Study the drawing (mm; zero at the part's minimum x, y, z) and answer. Give positions to 0.01 mm unless a question says otherwise; leave off trailing zeros. Write each loop counter-clockwise with the first axis right and the second up, starting at its lowest first coordinate (ties: lowest second). Pieces come first, ordered by that corner, then holes. Notation, with made-up numbers: (-19.75, 72) -> (-10.75, 72) arc R18 ccw to (-10.75, 104) -> close; hole circle Ø6 at (-35, -25.75). An arc over 180 degrees is marked (long way). Use CSV: the item, a comma, the result in double quotes. Start each with the question number.
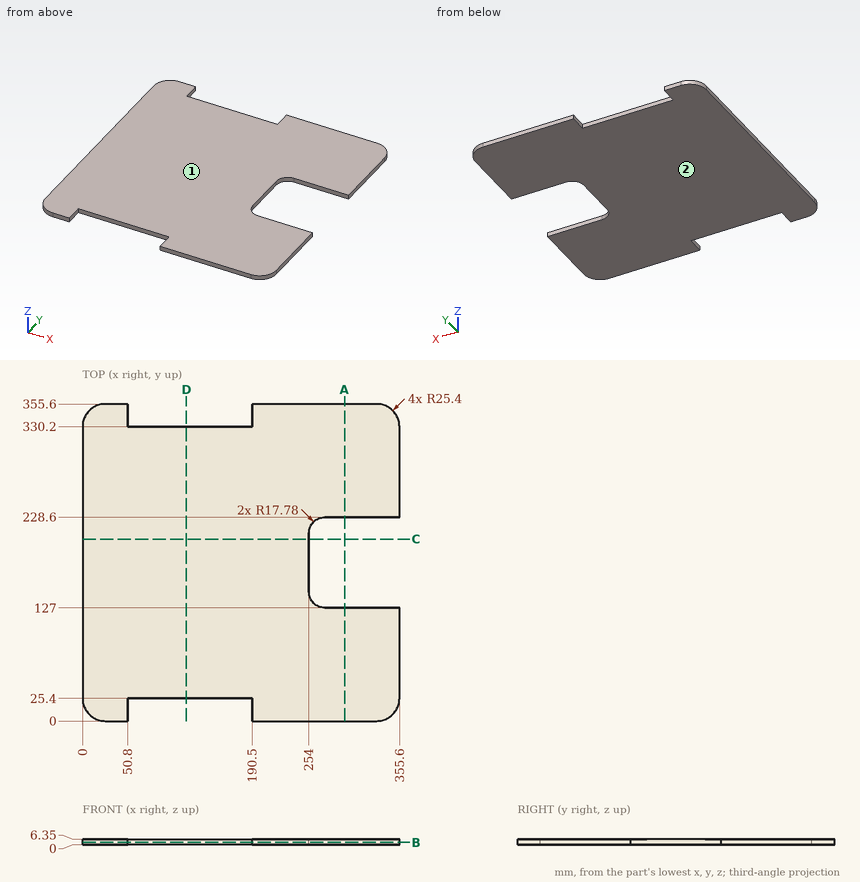
Q1. Section B-B on z = 2.5 is taken. Give the vertices of the cut face in (x, y).
Q2. Straight lines are drawn through the part: L1, parallel to Y at x = 284, z = 5.25; L2, parallel to Y at x = 88, z = 0.5; L3, parallel to X at y = 182.5, z = 4. For each, find the intervals that lie inside material, in ascending order.
Q3. Section D-D on x = 116.5 is taken. Give the vertices of the cut face in (y, z).
Q4. Flat-ended cylindrical pins translate along their axes: pin 1 Ø3 at (y, z) = (13, 3) entering from +X; pin 2 Ø1.9 at (y, z) = (342, 2.5) entering from +X; pin 3 Ø1 at (x, z) = (84, 3.5) entering from +Y. Find the tip coordinate at first contact, or state that the pin passes through.
Q5. Section A-A on x = 294 is taken. Give the vertices of the cut face in (y, z).
Q6. The mould has two halves that part along Z. Classify the marked faces 1 and 2: +Z half, -Z half, draft (parallel to the pull), parting line (faces both ways), or undercut.
Q7. Section C-C on y = 204 is taken. Give the vertices of the cut face in (x, z).
Output:
1,outline,"(0, 25.4) arc R25.4 ccw to (25.4, 0) -> (50.8, 0) -> (50.8, 25.4) -> (190.5, 25.4) -> (190.5, 0) -> (330.2, 0) arc R25.4 ccw to (355.6, 25.4) -> (355.6, 127) -> (271.78, 127) arc R17.78 cw to (254, 144.78) -> (254, 210.82) arc R17.78 cw to (271.78, 228.6) -> (355.6, 228.6) -> (355.6, 330.2) arc R25.4 ccw to (330.2, 355.6) -> (190.5, 355.6) -> (190.5, 330.2) -> (50.8, 330.2) -> (50.8, 355.6) -> (25.4, 355.6) arc R25.4 ccw to (0, 330.2) -> close"
2,L1,"0 to 127, 228.6 to 355.6"
2,L2,"25.4 to 330.2"
2,L3,"0 to 254"
3,outline,"(25.4, 0) -> (330.2, 0) -> (330.2, 6.35) -> (25.4, 6.35) -> close"
4,pin 1,"x = 353.14"
4,pin 2,"x = 353.17"
4,pin 3,"y = 330.2"
5,outline,"(0, 0) -> (127, 0) -> (127, 6.35) -> (0, 6.35) -> close; (228.6, 0) -> (355.6, 0) -> (355.6, 6.35) -> (228.6, 6.35) -> close"
6,face 1,"+Z half"
6,face 2,"-Z half"
7,outline,"(0, 0) -> (254, 0) -> (254, 6.35) -> (0, 6.35) -> close"
